```python
from build123d import *

# Parameters (mm, degrees)
F1_DEPTH  = 85
F2_W      = 145
F2_H      = 31
F3_DEPTH  = 82
F5_DEPTH  = 3
F6_R      = 36.5
F7_DEPTH  = 25
F8_W      = 150
F8_H      = 79
F9_DEPTH  = 25
F12_R     = 39.5
F11_R     = 22.5
F15_R     = 19.5
F16_R     = 36.5
F18_R     = 14.9183969034
F19_DEPTH = 25
F20_R     = 17.7986384492


with BuildPart() as f1:
    # F0 (on Front) → F1 (new body)
    with BuildSketch(Plane.XZ):
        with BuildLine():
            Line((53.6785274744, 17.5), (-77, 17.5))
            ThreePointArc((-77, 17.5), (-94.5, 0), (-77, -17.5))
            Line((-77, -17.5), (107, -17.5))
            Line((107, -17.5), (115.9520000219, -17.5))
            ThreePointArc((115.9520000219, -17.5), (120.1181090792, -1.0918428156), (118.9363524318, 15.7956536859))
            ThreePointArc((118.9363524318, 15.7956536859), (113.4877587414, 29.3800706908), (107, 42.5))
            ThreePointArc((107, 42.5), (92, 52.605015692), (77, 42.5))
            ThreePointArc((77, 42.5), (68.2201693479, 27.312521558), (53.6785274744, 17.5))
        make_face()
    extrude(amount=F1_DEPTH)

    # F2 (on face) → F3 (cut)
    with BuildSketch(Plane.XZ.offset(85)):
        Rectangle(F2_W, F2_H)
        with BuildLine():
            ThreePointArc((72.5, -15.5), (88, 0), (72.5, 15.5))
            Line((72.5, 15.5), (72.5, -15.5))
        make_face()
        with BuildLine():
            Line((-72.5, -15.5), (-72.5, 15.5))
            ThreePointArc((-72.5, 15.5), (-88, 0), (-72.5, -15.5))
        make_face()
    extrude(amount=-F3_DEPTH, mode=Mode.SUBTRACT)

    # F4 (on face) → F5 (join)
    with BuildSketch(Plane.XZ.offset(85)):
        Polygon((-80.3302004933, 15.8144365996), (-89.8194238544, 7.0904721506), (-91.0138636827, 2.9792727437), (-88.2837101817, -7.9413596541), (-85.0075185299, -14.220722951), (-77, -16.4173003286), (74.3856430054, -16.4173003286), (83.1666067243, -15.5), (93.1773036718, -10.9323309734), (95.8332046866, 5.4116621614), (83.1666067243, 16.6404508054), (67.7867159247, 16.6404508054), (-69.6145296097, 16.6404508054), align=None)
    extrude(amount=-F5_DEPTH)

    # F6 (on face) → F7 (cut)
    with BuildSketch(Plane.XY.offset(17.5)):
        with Locations((0, -42.5)):
            Circle(F6_R)
    extrude(amount=-F7_DEPTH, mode=Mode.SUBTRACT)

    # F8 (on face) → F9 (cut)
    with BuildSketch(Plane(origin=(0, 0, -17.5), x_dir=(1, 0, 0), z_dir=(0, 0, -1))):
        with Locations((0, 42.5)):
            Rectangle(F8_W, F8_H)
    extrude(amount=-F9_DEPTH, mode=Mode.SUBTRACT)

    # F12 (on face) → F13 section 0
    with BuildSketch(Plane.XY.offset(17.5)):
        with Locations((0, -42.5)):
            Circle(F12_R)
    # F11 (on offset) → F13 section 1
    with BuildSketch(Plane.XY.offset(62.5)):
        with Locations((0, -42.5)):
            Circle(F11_R)
    loft()

    # F15 (on offset) → F17 section 0
    with BuildSketch(Plane.XY.offset(60.5)):
        with Locations((0, -42.5)):
            Circle(F15_R)
    # F16 (on face) → F17 section 1
    with BuildSketch(Plane(origin=(0, 0, 17.5), x_dir=(1, 0, 0), z_dir=(0, 0, -1))):
        with Locations((0, 42.5)):
            Circle(F16_R)
    loft(mode=Mode.SUBTRACT)

    # F18 (on face) → F19 (cut)
    with BuildSketch(Plane.XY.offset(62.5)):
        with Locations((0, -42.5)):
            Circle(F18_R)
    extrude(amount=-F19_DEPTH, mode=Mode.SUBTRACT)

    # F20
    f20_edges = [f1.edges().sort_by_distance(p)[0] for p in [
        (115.952, -42.5, -17.5),
    ]]
    fillet(f20_edges, radius=F20_R)


solid = f1.part
```
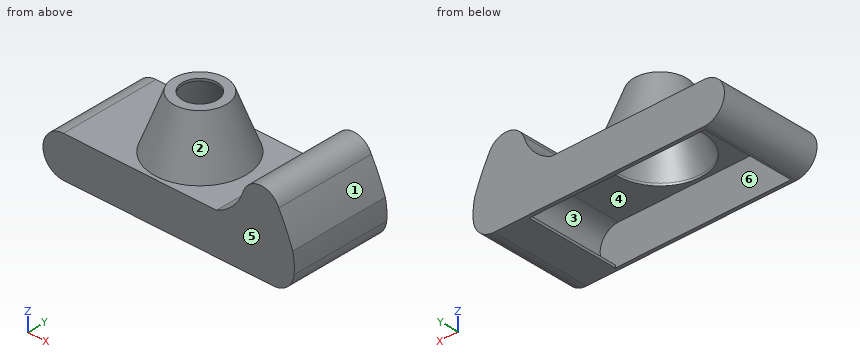
Read the model definition and answer for the solid it produces. Units are mm, in the model's axes. Face numbers are marked on the shaded views. A direction names the side the tool comes from. Give positions to 0.01 mm unless a question says otherwise; leave off trailing zeros. Write each loop counter-clockwise with the first axis right and the second up, starting at its lowest first coordinate (ties: lowest second). Pieces come first, ordered by that corner, then holes. Notation, with made-up numbers: (5, 82.25) - (26, 82.25) arc R36 ccw to (26, 117.25) - close; hole circle Ø1 at (-17.75, 25). An arc over 180 degrees is marked (long way). Write item = value, one per line. Start each with the question number.
Item 1: Find the intervals of material crossed by probe 1 along Y at (x, z) = (-5, -13); probe 2 along X at (y, z) = (-35.5, 24); probe 3 along X at (y, z) = (-40, 30), in increasing order. Write a range as [from, to].
Item 2: Find section A-A (x = 0). Give the vertices of the cut face in (y, z), then the cut area to 3 significant figures.
Item 3: Find section C-C (z = -11). Give the vertices of the cut face in (x, y), then the cut area to 3 significant figures.
Item 4: A tool of negligible diameter and unlimited length cuts with its end or side. For the marked faces 5 and 6, from which of +Z, -Z, +X, -X, +Y, -Y can it reach the whole face along a straight path? Write none if from no direction.
Item 5: The mould has two halves that part along Y. Classify the marked faces 1, 2, 3 and 4: +Y half, -Y half, draft (parallel to the pull), parting line (faces both ways), or undercut.
Item 6: Each of these flat-tipped pins is pushed along its axis until it touches: P1, Ø1.5, axis at x = -40.5, y = -60, coming from the -Z side; P2, Ø1.8, axis at y = -29.5, z = -16, coming from the +X side; P3, Ø18, axis at x = 0, y = -42.5, coming from the -Z side; P4, Ø10, axis at y = -23, z = 30.5, coming from the -X side. Where does it stop, or does it pass through?
Item 7: Find section B-B (z = 37). Give the vertices of the cut face in (x, y).
Response:
q1.probe_1 = [-85, -82], [-3, 0]
q1.probe_2 = [-36.38, -33.2], [33.2, 36.38], [64.72, 115.79]
q1.probe_3 = [-34.69, -31.46], [31.46, 34.69], [70.51, 113.21]
q2.outline = (-85, -17.5) - (-82, -17.5) - (-82, 15.5) - (-79, 15.5) - (-79, 17.5) - (-62, 60.5) - (-57.42, 60.5) - (-57.42, 62.5) - (-65, 62.5) - (-82, 17.5) - (-85, 17.5) - close; (-27.58, 60.5) - (-23, 60.5) - (-6, 17.5) - (-6, 15.5) - (-3, 15.5) - (-3, -17.5) - (0, -17.5) - (0, 17.5) - (-3, 17.5) - (-20, 62.5) - (-27.58, 62.5) - close
q2.area = 544 mm²
q3.outline = (-90.61, -85) - (116.12, -85) - (116.12, 0) - (-90.61, 0) - close; hole (-83.42, -82) - (83.42, -82) - (83.42, -3) - (-83.42, -3) - close
q3.area = 4,390 mm²
q4.face_5 = +Z, -Z, +X, -X, -Y
q4.face_6 = none
q5.face_1 = draft
q5.face_2 = parting line
q5.face_3 = undercut
q5.face_4 = undercut
q6.P1 = 15.5
q6.P2 = 111.3
q6.P3 = through
q6.P4 = -32.19
q7.outline = circle Ø64.27 at (0, -42.5); (74.85, -85) - (109.87, -85) - (109.87, 0) - (74.85, 0) - close; hole circle Ø57.58 at (0, -42.5)
